Source: CAD feature listing. Evaluate the final solid. Frame: model axes, mm. A direction names the side the tool comes from. Give positions to 0.01 mm unless a question says otherwise; leave off trailing zeros. Write each loop counter-clockwise with the first axis right and the second up, starting at its lowest first coordinate (ties: lowest second). Pieces come first, ordered by that corner, then holes.
```python
from build123d import *

# Parameters (mm, degrees)
SKETCH_1_W                   = 50
SKETCH_1_H                   = 50
SKETCH_1_W_2                 = 32.1
SKETCH_1_H_2                 = 32.1
EXTRUDE_1_DEPTH              = 8
CHAMFER_1_SIZE               = 10
CHAMFER_2_SIZE               = 6
HOLE_WIZARD_M3_1_D           = 3.2
HOLE_WIZARD_M3_1_CBORE_D     = 6
HOLE_WIZARD_M3_1_CBORE_DEPTH = 3.4
HOLE_WIZARD_M3_2_D           = 3.2
HOLE_WIZARD_M3_2_DEPTH       = 8.95
HOLE_WIZARD_M3_2_CBORE_D     = 6
HOLE_WIZARD_M3_2_CBORE_DEPTH = 3.4
HOLE_WIZARD_M3_3_D           = 3.2
HOLE_WIZARD_M3_3_DEPTH       = 8.95
HOLE_WIZARD_M3_3_CBORE_D     = 6
HOLE_WIZARD_M3_3_CBORE_DEPTH = 3.4
HOLE_WIZARD_M3_4_D           = 3.2
HOLE_WIZARD_M3_4_CBORE_D     = 6
HOLE_WIZARD_M3_4_CBORE_DEPTH = 3.4
HOLE_START                   = -25
HOLE_WIZARD_M3_5_OUTLINE_R   = 3
HOLE_WIZARD_M3_5_DEPTH       = 3.4
HOLE_START_2                 = -21.6
HOLE_WIZARD_M3_5_2_OUTLINE_R = 1.6
HOLE_WIZARD_M3_5_2_DEPTH     = 5.55
FILLET_1_R                   = 1
CHAMFER_4_SIZE               = 1


# Read off the part's stored shape, not the designer's step: M3 六角圆柱头螺钉的柱形沉头孔5
with BuildPart() as part:
    # 草图1 → 凸台-拉伸1 (new body)
    with BuildSketch(Plane(origin=(0, 0, 0), x_dir=(0, 0, -1), z_dir=(1, 0, 0))):
        Rectangle(SKETCH_1_W, SKETCH_1_H)
        Rectangle(SKETCH_1_W_2, SKETCH_1_H_2, mode=Mode.SUBTRACT)
    extrude(amount=EXTRUDE_1_DEPTH)

    # 倒角1
    chamfer_1_edges = [part.edges().sort_by_distance(p)[0] for p in [
        (4, -25, -25),
        (4, -25, 25),
        (4, 25, 25),
        (4, 25, -25),
    ]]
    chamfer(chamfer_1_edges, length=CHAMFER_1_SIZE)

    # 倒角2
    chamfer_2_edges = [part.edges().sort_by_distance(p)[0] for p in [
        (4, -16.05, -16.05),
        (4, 16.05, -16.05),
        (4, 16.05, 16.05),
        (4, -16.05, 16.05),
    ]]
    chamfer(chamfer_2_edges, length=CHAMFER_2_SIZE)

    # M3 六角圆柱头螺钉的柱形沉头孔1 (through all)
    with Locations(Plane(origin=(8, 0, 0), x_dir=(0, 0, -1), z_dir=(1, 0, 0))):
        with Locations((-13.959899742, 19.214153616), (13.959899742, 19.214153616), (19.214153616, -13.959899742), (-13.959899742, -19.214153616), (-19.214153616, 13.959899742), (19.214153616, 13.959899742), (13.959899742, -19.214153616), (-19.214153616, -13.959899742)):
            CounterBoreHole(HOLE_WIZARD_M3_1_D / 2, HOLE_WIZARD_M3_1_CBORE_D / 2, HOLE_WIZARD_M3_1_CBORE_DEPTH)

    # M3 六角圆柱头螺钉的柱形沉头孔2
    with Locations(Plane(origin=(0, 25, 0), x_dir=(1, 0, 0), z_dir=(0, 1, 0))):
        with Locations((4, 0)):
            CounterBoreHole(HOLE_WIZARD_M3_2_D / 2, HOLE_WIZARD_M3_2_CBORE_D / 2, HOLE_WIZARD_M3_2_CBORE_DEPTH, depth=HOLE_WIZARD_M3_2_DEPTH)

    # M3 六角圆柱头螺钉的柱形沉头孔3
    with Locations(Plane(origin=(0, 0, -25), x_dir=(-1, 0, 0), z_dir=(0, 0, -1))):
        with Locations((-4, 6), (-4, -6)):
            CounterBoreHole(HOLE_WIZARD_M3_3_D / 2, HOLE_WIZARD_M3_3_CBORE_D / 2, HOLE_WIZARD_M3_3_CBORE_DEPTH, depth=HOLE_WIZARD_M3_3_DEPTH)

    # M3 六角圆柱头螺钉的柱形沉头孔4 (through all)
    with Locations(Plane.XY.offset(25)):
        with Locations((4, -6), (4, 6)):
            CounterBoreHole(HOLE_WIZARD_M3_4_D / 2, HOLE_WIZARD_M3_4_CBORE_D / 2, HOLE_WIZARD_M3_4_CBORE_DEPTH)

    # M3 六角圆柱头螺钉的柱形沉头孔5 outline → M3 六角圆柱头螺钉的柱形沉头孔5 (cut)
    with BuildSketch(Plane(origin=(0, 0, 0), x_dir=(1, 0, 0), z_dir=(0, 1, 0)).offset(HOLE_START)):
        with Locations((4, 0)):
            Circle(HOLE_WIZARD_M3_5_OUTLINE_R)
    extrude(amount=HOLE_WIZARD_M3_5_DEPTH, mode=Mode.SUBTRACT)

    # Hole Wizard M3 _5 2 outline → Hole Wizard M3 _5 2 (cut)
    with BuildSketch(Plane(origin=(0, 0, 0), x_dir=(1, 0, 0), z_dir=(0, 1, 0)).offset(HOLE_START_2)):
        with Locations((4, 0)):
            Circle(HOLE_WIZARD_M3_5_2_OUTLINE_R)
    extrude(amount=HOLE_WIZARD_M3_5_2_DEPTH, mode=Mode.SUBTRACT)

    # 圆角1
    fillet_1_edges = [part.edges().sort_by_distance(p)[0] for p in [
        (4, -25, -15),
        (4, -25, 15),
        (4, 15, 25),
        (4, -15, 25),
        (4, 15, -25),
        (4, -15, -25),
        (4, 25, 15),
        (4, 25, -15),
    ]]
    fillet(fillet_1_edges, radius=FILLET_1_R)

    # 倒角4
    chamfer_4_edges = [part.edges().sort_by_distance(p)[0] for p in [
        (8, 25, 0),
        (0, 25, 0),
        (8, 0, 25),
        (8, -20, 20),
        (8, -25, 0),
        (8, -20, -20),
        (8, 0, -25),
        (8, 20, -20),
        (8, 20, 20),
        (8, -14.96846987, 24.923879533),
        (8, -24.923879533, 14.96846987),
        (8, -24.923879533, -14.96846987),
        (8, -14.96846987, -24.923879533),
        (8, 14.96846987, -24.923879533),
        (8, 24.923879533, -14.96846987),
        (8, 14.96846987, 24.923879533),
        (8, 24.923879533, 14.96846987),
        (0, 20, 20),
        (0, -25, 0),
        (0, -20, 20),
        (0, 0, 25),
        (0, 20, -20),
        (0, 0, -25),
        (0, -20, -20),
        (0, -14.96846987, 24.923879533),
        (0, -24.923879533, 14.96846987),
        (0, -24.923879533, -14.96846987),
        (0, -14.96846987, -24.923879533),
        (0, 14.96846987, -24.923879533),
        (0, 24.923879533, -14.96846987),
        (0, 14.96846987, 24.923879533),
        (0, 24.923879533, 14.96846987),
        (0, 0, 16.05),
        (8, 0, 16.05),
        (0, -16.05, 0),
        (8, -16.05, 0),
        (0, 0, -16.05),
        (8, 0, -16.05),
        (0, 16.05, 0),
        (8, 16.05, 0),
        (0, -13.05, 13.05),
        (8, -13.05, 13.05),
        (0, -13.05, -13.05),
        (8, -13.05, -13.05),
        (0, 13.05, -13.05),
        (8, 13.05, -13.05),
        (0, 13.05, 13.05),
        (8, 13.05, 13.05),
    ]]
    chamfer(chamfer_4_edges, length=CHAMFER_4_SIZE - 0.0001)  # a hair under: the kernel refuses the full size


solid = part.part
```
1. Cut plane B-B, the plane z = 9. Return the cut outline in (x, y), then the cut area to 3 significant figures.
2. Cut plane A-A, the plane y = 6. State how many separate pieces and enclosed holes the cut face has, then the cut area to 3 significant figures.
3. Line query: L1, parallel to Y at x = 2.75, z = -3; L2, parallel to Y at x = 5.5, z = 1.5. Output: solid intervals per line, ascending.
4. Access query for faces 5 (the flat face through (4, -20, 20)), 6 (the flat face through (2.7, 4.7, -21.6)), 7 (the flat face through (0.51, 13.44, 13.35)), 8 (the flat face through (4, 13, 13.1)), 9 (the cylindrical face through (6.324, 18.065, 11.189)). Directions: +Z, -Z, +X, -X, +Y, -Y. A direction counts if a zero-diameter tool reaches every point of the face in a straight line with its end or side. Return the directions, or none.
5. Contact query for flat-ended pins moving along their axis: P1, Ø2.5, axis at y = 13.96, z = -19.21, coming from the +X side; P2, Ø4, axis at x = 4, y = -6, coming from the -Z side; P3, Ø3.5, axis at y = -19.21, z = -13.96, coming from the +X side; P4, Ø1.8, axis at x = 4, z = 1, coming from the -Y side. Output: stop coordinate, or through.
6. Cut plane D-D, the plane z = -19. Return the cut outline in (x, y), then the cut area to 3 significant figures.
7. Mould query, pull axis Y, two halves, no side actions, for faces 1 (the flat face through (0.51, -19.59, -19.72)), 2 (the flat face through (4.6, -21, -15)), 3 (the flat face through (4, 0, -25)), 4 (the flat face through (2, 16.05, 0)). Classes: +Y half, -Y half, draft (parallel to the pull), parting line (faces both ways), or undercut.
Response values:
1. outline: (0, -24) - (1, -25) - (7, -25) - (8, -24) - (8, -17.05) - (7, -16.05) - (1, -16.05) - (0, -17.05) - close; (0, 17.05) - (1, 16.05) - (7, 16.05) - (8, 17.05) - (8, 24) - (7, 25) - (1, 25) - (0, 24) - close
1. area: 139 mm2
2. separate pieces: 4
2. enclosed holes: 0
2. area: 62.9 mm2
3. L1: y = -25 to -16.05, 16.05 to 25
3. L2: y = -21.6 to -16.05, 16.05 to 21.6
4. face 5: +Z, +X, -X, -Y
4. face 6: -Z
4. face 7: -X
4. face 8: +X, -X
4. face 9: +X
5. P1: passes through
5. P2: stops at z = -21.6
5. P3: stops at x = 4.6
5. P4: stops at y = -21.6
6. outline: (0, -19.59) - (1, -21) - (7, -21) - (8, -19.59) - (8, -16.95) - (4.6, -16.95) - (4.6, -15.55) - (0, -15.55) - close; (0, -12.37) - (4.6, -12.37) - (4.6, -10.97) - (8, -10.97) - (8, 10.97) - (4.6, 10.97) - (4.6, 12.37) - (0, 12.37) - close; (0, 15.55) - (4.6, 15.55) - (4.6, 16.95) - (8, 16.95) - (8, 19.59) - (7, 21) - (1, 21) - (0, 19.59) - close; hole circle Ø3.2 at (4, -6); hole circle Ø3.2 at (4, 6)
6. area: 247 mm2
7. face 1: -Y half
7. face 2: undercut
7. face 3: draft
7. face 4: undercut
